Build history of the part. All positions in model axes, mm. A direction names the side the tool comes from. Round coordinates to 2 decimals unless told otherwise and drop trailing zeros. Order: outer loops, then holes, each group sorted by start corner. A loop starts at its lowest first (then second) coordinate and runs counter-clockwise, first axis right, second up. Notation, with made-up numbers: M 89.25,70.25 L 119.25,70.25 A27 cw 119.25,102.25 Z; hole C -22,25 d1. An arc over 180 degrees is marked long. One line per item, written item: value. Start each with the question number.
Item 1: Band-saw the part on B-B, the plane x = 100. Write the cut outline in (y, z).
Item 2: Two-plate mould, pull along Z, no slides. Class faces 3 (the flat face through (99.9, 20, -10.2)), 4 (the cylindrical face through (90, 10, 0)), 5 (the flat face through (44, 5, -7.5)): +Z half, -Z half, draft (parallel to the pull), parting line (faces both ways), or undercut.
Item 3: Pin check, flat tips, straight feed: pin 1 (5 mm diameter, centred on x = 31, z = 9.5, fed in from -Y); pin 2 (11 mm diameter, centred on x = 41.5, y = 5, fed in from +Z); pin 3 (3 mm diameter, centred on y = 8, z = -3, fed in from -X); pin 4 (2 mm diameter, centred on x = 43, y = 5.5, fed in from -Z). Stop position of each tip, or through.
Item 4: Tool access for faces 1 (the cylindrical face through (-7.5, 4.93, 0.16)), 2 (the flat face through (46, 5, 7.5)): list every direction of +Z, -Z, +X, -X, +Y, -Y with a clear straight run to the whole face (end or side of a thin tool).
Item 5: Probe L1, parallel to X at y = 5, z = 0; L2, parallel to Z at x = 0, y = 5; L3, parallel to Z at x = 99.5, y = 4.75. List the from-to ranges inside material, lowest first.
Item 6: Band-saw the part on D-D, the plane y = 8.75. Write the cut outline in (x, z), then the cut area to 3 significant figures.
Item 7: Band-saw the part on A-A, the plane z = 0. Write the cut outline in (x, y).
Item 8: Band-saw the part on C-C, the plane z = 5.75. Write the cut outline in (x, y).
```python
from build123d import *

# Parameters (mm, degrees)
SKETCH2_R           = 2
SKETCH2_R_2         = 2.5
BOSS_EXTRUDE1_DEPTH = 10
SKETCH3_R           = 12.5
BOSS_EXTRUDE3_DEPTH = 20
CUT_EXTRUDE1_REACH  = 22
SKETCH4_R           = 10


with BuildPart() as part:
    # Sketch2 → Boss-Extrude1 (new body)
    with BuildSketch(Plane(origin=(0, 0, 0), x_dir=(1, 0, 0), z_dir=(0, 1, 0))):
        with BuildLine():
            Line((0, 7.5), (100, 7.5))
            ThreePointArc((100, 7.5), (107.5, 0), (100, -7.5))
            Line((100, -7.5), (0, -7.5))
            ThreePointArc((0, -7.5), (-7.5, 0), (0, 7.5))
        make_face()
        Circle(SKETCH2_R, mode=Mode.SUBTRACT)
        with Locations((100, 0)):
            Circle(SKETCH2_R_2, mode=Mode.SUBTRACT)
    extrude(amount=BOSS_EXTRUDE1_DEPTH)

    # Sketch3 → Boss-Extrude3 (add)
    with BuildSketch(Plane(origin=(0, 0, 0), x_dir=(1, 0, 0), z_dir=(0, 1, 0))):
        with Locations((100, 0)):
            Circle(SKETCH3_R)
    extrude(amount=BOSS_EXTRUDE3_DEPTH)

    # Sketch4 → Cut-Extrude1 (cut, up to next)
    with BuildSketch(Plane(origin=(0, 20, 0), x_dir=(1, 0, 0), z_dir=(0, 1, 0)), mode=Mode.PRIVATE) as cut_extrude1_sk1:
        with Locations((100, 0)):
            Circle(SKETCH4_R)
    cut_extrude1_tool1 = extrude(cut_extrude1_sk1.sketch, amount=-CUT_EXTRUDE1_REACH, mode=Mode.PRIVATE) & part.part
    add(cut_extrude1_tool1.solids().sort_by_distance((100, 20, 0))[0], mode=Mode.SUBTRACT)


solid = part.part
```
Output:
1. outline: M 0,-12.5 L 20,-12.5 L 20,-10 L 0,-10 Z; M 0,10 L 20,10 L 20,12.5 L 0,12.5 Z
2. face 3: draft
2. face 4: undercut
2. face 5: -Z half
3. pin 1: stops at y = 0
3. pin 2: stops at z = 7.5
3. pin 3: stops at x = -7.35
3. pin 4: stops at z = -7.5
4. face 1: -X, +Y, -Y
4. face 2: +Z, -X, +Y, -Y
5. L1: x = -7.5 to -2, 2 to 90, 110 to 112.5
5. L2: z = -7.5 to -2, 2 to 7.5
5. L3: z = -12.49 to -9.99, 9.99 to 12.49
6. outline: M 0,-7.5 L 90,-7.5 A12.5 ccw long 90,7.5 L 0,7.5 A7.5 ccw Z; hole C 0,0 d4; hole C 100,0 d20
6. area: 1,580 mm²
7. outline: M -7.5,0 L -2,0 L -2,10 L -7.5,10 Z; M 2,0 L 90,0 L 90,20 L 87.5,20 L 87.5,10 L 2,10 Z; M 110,0 L 112.5,0 L 112.5,20 L 110,20 Z
8. outline: M -4.82,0 L 91.82,0 L 91.82,20 L 88.9,20 L 88.9,10 L -4.82,10 Z; M 108.18,0 L 111.1,0 L 111.1,20 L 108.18,20 Z
